The model under review builds one solid part; all positions refer to its coordinate system, in mm. A direction names the side the tool comes from. Round coordinates to 2 decimals unless told otherwise and drop trailing zeros. Order: outer loops, then holes, each group sorted by start corner. A loop starts at its lowest first (then second) coordinate and runs counter-clockwise, first axis right, second up.
1) To check wall thickness, follow L1, parallel to X at y = 9.5, z = 0.4; L2, parallel to X at y = 13, z = 0.5; L3, parallel to Y at x = -35, z = 0.2. State the ranges of each line that lie inside material, in increasing order.
2) Consider section C-C (z = 0.5). Give the boundary of the cut face in (x, y).
3) Consider section D-D (y = 13.5). Give the boundary of the cut face in (x, z).
4) Machinability: for faces 1 (the face through (-1, 0, 0)), 2 (the face through (-15.004, -15.177, 0.394)), which of the approach directions +Z, -Z, +X, -X, +Y, -Y give a long, thin tool a straight path to every point of the face, cutting with its end or side? Answer none if there is none.
5) Mouldability with a two-part tool opening along X and no side actions: class faces 3 (the face through (14.834, -15.177, 0.394)), 4 (the face through (-1, 0, 0.8)) as pulls with the +X half, pulls with the -X half, needs draft (parallel to the pull), parting line crosses it, or undercut.
6) Consider section A-A (y = -7.5). Give the boundary of the cut face in (x, z).
7) Consider section B-B (x = -30). Give the boundary of the cut face in (y, z), then the cut area to 3 significant figures.
from build123d import *

# Parameters (mm, degrees)
SKETCH_1_W      = 105.64042879
SKETCH_1_H      = 41.546296754
SKETCH_1_R      = 2.8
EXTRUDE_2_DEPTH = 0.8


with BuildPart() as part:
    # Эскиз1 → Бобышка-Вытянуть2 (new body)
    with BuildSketch(Plane.XY):
        with Locations((0.083446622, -0.02774538)):
            Rectangle(SKETCH_1_W, SKETCH_1_H)
        with Locations((0.083446622, -15.17774538)):
            Circle(SKETCH_1_R, mode=Mode.SUBTRACT)
        with BuildLine():
            Line((-49.635877413, 10.77725462), (-49.635877413, -10.83274538))
            ThreePointArc((-49.635877413, -10.83274538), (-38.735877413, -15.17774538), (-27.835877413, -10.83274538))
            Line((-27.835877413, -10.83274538), (-27.835877413, 10.77725462))
            ThreePointArc((-27.835877413, 10.77725462), (-38.735877413, 15.12225462), (-49.635877413, 10.77725462))
        make_face(mode=Mode.SUBTRACT)
        with BuildLine():
            Line((-25.735877413, 10.77725462), (-25.735877413, -10.83274538))
            ThreePointArc((-25.735877413, -10.83274538), (-14.835877413, -15.17774538), (-3.935877413, -10.83274538))
            Line((-3.935877413, -10.83274538), (-3.935877413, 10.77725462))
            ThreePointArc((-3.935877413, 10.77725462), (-14.835877413, 15.12225462), (-25.735877413, 10.77725462))
        make_face(mode=Mode.SUBTRACT)
        with BuildLine():
            Line((4.102770658, 10.77725462), (4.102770658, -10.83274538))
            ThreePointArc((4.102770658, -10.83274538), (15.002770658, -15.17774538), (25.902770658, -10.83274538))
            Line((25.902770658, -10.83274538), (25.902770658, 10.77725462))
            ThreePointArc((25.902770658, 10.77725462), (15.002770658, 15.12225462), (4.102770658, 10.77725462))
        make_face(mode=Mode.SUBTRACT)
        with BuildLine():
            Line((28.002770658, 10.77725462), (28.002770658, -10.83274538))
            ThreePointArc((28.002770658, -10.83274538), (38.902770658, -15.17774538), (49.802770658, -10.83274538))
            Line((49.802770658, -10.83274538), (49.802770658, 10.77725462))
            ThreePointArc((49.802770658, 10.77725462), (38.902770658, 15.12225462), (28.002770658, 10.77725462))
        make_face(mode=Mode.SUBTRACT)
    extrude(amount=EXTRUDE_2_DEPTH)


solid = part.part
Answer below:
1. L1: x = -52.74 to -49.64, -27.84 to -25.74, -3.94 to 4.1, 25.9 to 28, 49.8 to 52.9
1. L2: x = -52.74 to -46.66, -30.81 to -22.76, -6.91 to 7.08, 22.92 to 30.98, 46.82 to 52.9
1. L3: y = -20.8 to -14.73, 14.68 to 20.75
2. outline: (-52.74, -20.8) - (52.9, -20.8) - (52.9, 20.75) - (-52.74, 20.75) - close; hole (-49.64, -10.83) arc R15.84 ccw to (-27.84, -10.83) - (-27.84, 10.78) arc R15.84 ccw to (-49.64, 10.78) - close; hole (-25.74, -10.83) arc R15.84 ccw to (-3.94, -10.83) - (-3.94, 10.78) arc R15.84 ccw to (-25.74, 10.78) - close; hole circle Ø5.6 at (0.08, -15.18); hole (4.1, -10.83) arc R15.84 ccw to (25.9, -10.83) - (25.9, 10.78) arc R15.84 ccw to (4.1, 10.78) - close; hole (28, -10.83) arc R15.84 ccw to (49.8, -10.83) - (49.8, 10.78) arc R15.84 ccw to (28, 10.78) - close
3. outline: (-52.74, 0) - (-45.72, 0) - (-45.72, 0.8) - (-52.74, 0.8) - close; (-31.75, 0) - (-21.82, 0) - (-21.82, 0.8) - (-31.75, 0.8) - close; (-7.85, 0) - (8.02, 0) - (8.02, 0.8) - (-7.85, 0.8) - close; (21.99, 0) - (31.92, 0) - (31.92, 0.8) - (21.99, 0.8) - close; (45.89, 0) - (52.9, 0) - (52.9, 0.8) - (45.89, 0.8) - close
4. face 1: -Z, +X, -X, +Y, -Y
4. face 2: +Z, -Z
5. face 3: undercut
5. face 4: needs draft
6. outline: (-52.74, 0) - (-49.64, 0) - (-49.64, 0.8) - (-52.74, 0.8) - close; (-27.84, 0) - (-25.74, 0) - (-25.74, 0.8) - (-27.84, 0.8) - close; (-3.94, 0) - (4.1, 0) - (4.1, 0.8) - (-3.94, 0.8) - close; (25.9, 0) - (28, 0) - (28, 0.8) - (25.9, 0.8) - close; (49.8, 0) - (52.9, 0) - (52.9, 0.8) - (49.8, 0.8) - close
7. outline: (-20.8, 0) - (-12.55, 0) - (-12.55, 0.8) - (-20.8, 0.8) - close; (12.5, 0) - (20.75, 0) - (20.75, 0.8) - (12.5, 0.8) - close
7. area: 13.2 mm2
